Can you work these out from the model? Positions are in its coordinate system, mm. A direction names the side the tool comes from. Round coordinates to 2 decimals unless told otherwise and drop trailing zeros. Order: outer loops, then holes, each group sorted by start corner. A loop starts at its lowest first (then second) coordinate and runs counter-clockwise, first axis right, second up. Notation, with made-up numbers: M 48,15.25 L 73,15.25 A19 cw 73,19.25 Z; hole C 28.25,23.25 d9. An arc over 180 degrees is marked long. Answer as a JSON object with one key per item and string values. Group by question number.
Autodesk Inventor part; units mm, degrees
ref_plane "YZ Plane" through (0, 0, 0) normal (1, 0, 0) x (0, 1, 0)
ref_plane "XZ Plane" through (0, 0, 0) normal (0, 1, 0) x (-1, 0, 0)
ref_plane "XY Plane" through (0, 0, 0) normal (0, 0, 1) x (1, 0, 0)
sketch "Outer Diameter Sketch" plane through (0, 0, 0) normal (0, 1, 0) x (-1, 0, 0)
  line L0 (0, -28.0163) -> (0, 28.3344) construction
  line L1 (17.1062, 0) -> (-23.8822, 0) construction
  line L2 (3.4641, -6) -> (6.9282, 0)
  line L3 (6.9282, 0) -> (3.4641, 6)
  line L4 (3.4641, 6) -> (-3.4641, 6)
  line L5 (-3.4641, 6) -> (-6.9282, 0)
  line L6 (-6.9282, 0) -> (-3.4641, -6)
  line L7 (-3.4641, -6) -> (3.4641, -6)
  line L8 (0, -6) -> (0, 6) construction
  line L9 (-6.9282, 0) -> (6.9282, 0) construction
  point P0 (0, 0)
  dimension "d23" = 120
  dimension "d25" = 120
  dimension "d27" = 120
  dimension "d29" = 120
  dimension "d31" = 120
  dimension "d32" = 12
extrude "Outer Diameter Extrusion" add sketch "Outer Diameter Sketch" along normal mid plane 112
sketch "Sketch2" plane through (0, 0, 0) normal (1, 0, 0) x (0, 1, 0)
  circle A0 centre (0, 0) radius 4
  line L0 (-56, 0) -> (0, 0) construction
  line L1 (0, 0) -> (56, 0) construction
  circle A1 centre (15.6667, 0) radius 4
  circle A2 centre (31.3333, 0) radius 4
  circle A3 centre (47, 0) radius 4
  circle A4 centre (-15.6667, 0) radius 4
  circle A5 centre (0, 0) radius 4
  circle A6 centre (15.6667, 0) radius 4
  circle A7 centre (31.3333, 0) radius 4
  circle A8 centre (-31.3333, 0) radius 4
  circle A9 centre (-15.6667, 0) radius 4
  circle A10 centre (0, 0) radius 4
  circle A11 centre (15.6667, 0) radius 4
  circle A12 centre (-47, 0) radius 4
  circle A13 centre (-31.3333, 0) radius 4
  circle A14 centre (-15.6667, 0) radius 4
  circle A15 centre (0, 0) radius 4
  dimension "d3" = 8
  dimension "d5" = 112
  dimension "d8" = 15.6667
  dimension "d11" = 15.6667
extrude "Extrusion2" add sketch "Sketch2" along normal mid plane 32
sketch "Sketch3" plane through (0, -56, 0) normal (0, -1, 0) x (1, 0, 0)
  line L0 (1.55, -2.6847) -> (-1.55, -2.6847)
  line L1 (-1.55, -2.6847) -> (-3.1, 0)
  line L2 (-3.1, 0) -> (-1.55, 2.6847)
  line L3 (-1.55, 2.6847) -> (1.55, 2.6847)
  line L4 (1.55, 2.6847) -> (3.1, 0)
  line L5 (3.1, 0) -> (1.55, -2.6847)
  line L6 (3.1, 0) -> (-3.1, 0) construction
  line L7 (0, 2.6847) -> (0, -2.6847) construction
  line L8 (10.3659, 0) -> (-11.745, 0) construction
  line L9 (0, -9.4896) -> (0, 9.303) construction
  point P0 (0, 0)
  dimension "d33" = 3.1
  dimension "d34" = 3.1
  dimension "d35" = 120
  dimension "d36" = 3.1
  dimension "d37" = 120
  dimension "d38" = 3.1
  dimension "d39" = 120
  dimension "d40" = 3.1
  dimension "d41" = 120
extrude "Extrusion3" cut sketch "Sketch3" against normal up to surface (112 mm away)
equation "\"d1\" = outL"
equation "\"d3\" = pegD"
equation "\"d5\" = outL"
equation "\"d14\" = pegL + 2 * outD"
equation "\"d33\" = inhexSL"
equation "\"d34\" = inhexSL"
equation "\"d36\" = inhexSL"
equation "\"d38\" = inhexSL"
equation "\"d40\" = inhexSL"
equation "\"d42\" = pegL + 2 * outD"
equation "\"outD\" = 12"
equation "\"inhexSL\" = 3.1"
equation "\"outL\" = 112"
equation "\"pegL\" = 8"
equation "\"pegD\" = 8"
equation "\"outhexSL\" = 5"
properties part number "Peg Spinner"
Item 1: I need wall thicknesses on line 1 (Z direction, x = 8, y = -47); line 2 (X direction, y = -34, z = 0.75); line 3 (Z direction, x = -1, y = 36). Which ranges of each line are inside material? Lowest first, please.
Item 2: Suppose I cut it at C-C, the plane y = -18. Write out the boundary of the cut face in (x, z), and give its area (3 significant figures).
Item 3: I'm going to push flat-ended pins straight in: pin 1 Ø2 at (x, z) = (8.5, -4.5) entering from +Y; pin 2 Ø8 at (x, y) = (11, -8) entering from -Z. Where does each tip first touch, or does it pass through?
Item 4: Suppose I cut it at B-B, the plane y = -40. Write out the boundary of the cut face in (x, z), and give its area (3 significant figures).
Item 5: Suppose I cut it at A-A, the plane x = 8. Write out the boundary of the cut face in (y, z).
Item 6: On a 3-axis mill with a long thin cutter (end or side, diameter ignored), from which of +Z, -Z, +X, -X, +Y, -Y can I reach the whole of each face in a straight line? I mean faces 3 (the face through (0, -1, -6)), 4 (the face through (0, -1, -2.685)), 5 (the face through (-10.226, 19.362, -1.532)), 6 (the face through (10.226, 50.815, -1.201)). Say none if no direction works.
Item 7: If we mould it in two halves opening along Y, with no side actions, what happens to faces 1 (the face through (10.23, -11.97, 1.53)), 2 (the face through (-16, 16, 0))? For each: +Y half, -Y half, draft (parallel to the pull), parting line (faces both ways), or undercut.
Computed:
{
 "1": {"line 1": "z = -4 to 4", "line 2": "x = -16 to -2.67, 2.67 to 16", "line 3": "z = -6 to -2.68, 2.68 to 6"},
 "2": {"outline": "M -16,-3.25 L -5.05,-3.25 L -3.46,-6 L 3.46,-6 L 5.05,-3.25 L 16,-3.25 L 16,3.25 L 5.05,3.25 L 3.46,6 L -3.46,6 L -5.05,3.25 L -16,3.25 Z; hole M -3.1,0 L -1.55,-2.68 L 1.55,-2.68 L 3.1,0 L 1.55,2.68 L -1.55,2.68 Z", "area": "230 mm^2"},
 "3": {"pin 1": "stops at y = 48.94", "pin 2": "stops at z = -1.6"},
 "4": {"outline": "M -6.93,0 L -3.46,-6 L 3.46,-6 L 6.93,0 L 3.46,6 L -3.46,6 Z; hole M -3.1,0 L -1.55,-2.68 L 1.55,-2.68 L 3.1,0 L 1.55,2.68 L -1.55,2.68 Z", "area": "99.7 mm^2"},
 "5": {"outline": "C -47,0 d8; C -31.33,0 d8; C -15.67,0 d8; C 0,0 d8; C 15.67,0 d8; C 31.33,0 d8; C 47,0 d8"},
 "6": {"face 3": "-Z, +X, -X, +Y, -Y", "face 4": "+Y, -Y", "face 5": "-X", "face 6": "+X"},
 "7": {"face 1": "undercut", "face 2": "draft"}
}
